```python
from build123d import *

# Parameters (mm, degrees)
FILLET1_R          = 0.1
SKETCH2_R          = 2.5
CUT_EXTRUDE1_DEPTH = 0.5


with BuildPart() as part:
    # Sketch1 → Revolve1 (revolve)
    with BuildSketch(Plane.XY, mode=Mode.PRIVATE) as revolve1_sk:
        Polygon((0, 0), (0, 1.2), (2.935572642, 1.2), (3, 0.463591927), (2.812696703, 0), align=None)
    revolve(revolve1_sk.sketch.rotate(Axis((0, 0, 0), (0, 1, 0)), 90), axis=Axis((0, 0, 0), (0, 1, 0)))

    # Fillet1
    fillet1_edges = [part.edges().sort_by_distance(p)[0] for p in [
        (0, 1.2, 2.935572642),
    ]]
    fillet(fillet1_edges, radius=FILLET1_R)

    # Sketch2 → Cut-Extrude1 (cut)
    with BuildSketch(Plane.XZ):
        with Locations(Location((0, 0, 0), (0, 0, 270))):
            Circle(SKETCH2_R)
    extrude(amount=-CUT_EXTRUDE1_DEPTH, mode=Mode.SUBTRACT)


solid = part.part
```
Part model, mm, in its own coordinate system. Round coordinates to 2 decimals unless told otherwise and drop trailing zeros. Order: outer loops, then holes, each group sorted by start corner. A loop starts at its lowest first (then second) coordinate and runs counter-clockwise, first axis right, second up. Notation, with made-up numbers: M 19.5,17.25 L 57.5,17.25 A10 cw 57.5,22.25 Z; hole C 68.5,11.25 d9. An arc over 180 degrees is marked long. Put each result on its own line as item: value. Start each with the question number.
1. Slice it at A-A on x = 0. List the corners of the cut face in (y, z).
2. Drop flat-ended pins along their axis: pin 1 (2.5 mm diameter, centred on x = -0.5, z = -1, fed in from -Y); pin 2 (1.5 mm diameter, centred on x = 1.5, z = 2, fed in from -Y). Give the stop position or say it passes through.
3. Slice it at B-B on z = 0. List the corners of the cut face in (x, y).
4. Two-plate mould, pull along X, no slides. Class faces 1 (the face through (0, 0.5, 0)), 2 (the face through (0, 1.2, 0)): +X half, -X half, draft (parallel to the pull), parting line (faces both ways), or undercut.
5. Drill centre lines: probe 1 along Y at (x, z) = (-0.85, 1.75); probe 2 along X at (y, z) = (0.25, -2); probe 3 along X at (y, z) = (0.4, 0). Where is each one in solid material? Low to high. Write a range as [from, to].
6. Slice it at C-C on y = 0.3. List the corners of the cut face in (x, z).
Findings:
1. outline: M 0,-2.81 L 0.46,-3 L 1.11,-2.94 A0.1 ccw 1.2,-2.84 L 1.2,2.84 A0.1 ccw 1.11,2.94 L 0.46,3 L 0,2.81 L 0,2.5 L 0.5,2.5 L 0.5,-2.5 L 0,-2.5 Z
2. pin 1: y = 0.5
2. pin 2: y = 0
3. outline: M -3,0.46 L -2.81,0 L -2.5,0 L -2.5,0.5 L 2.5,0.5 L 2.5,0 L 2.81,0 L 3,0.46 L 2.94,1.11 A0.1 ccw 2.84,1.2 L -2.84,1.2 A0.1 ccw -2.94,1.11 Z
4. face 1: undercut
4. face 2: draft
5. probe 1: [0.5, 1.2]
5. probe 2: [-2.12, -1.5], [1.5, 2.12]
5. probe 3: [-2.97, -2.5], [2.5, 2.97]
6. outline: C 0,0 d5.87; hole C 0,0 d5
